from build123d import *

# Parameters (mm, degrees)
F0_R     = 1.45
F1_DEPTH = 7.62
F2_R     = 1.877804
F3_DEPTH = 25.4
F5_W     = 7.426485
F5_H     = 4.44201
F6_DEPTH = 25.4


with BuildPart() as f1:
    # F0 (on Right) → F1 (new body)
    with BuildSketch(Plane.YZ):
        with Locations((0, 11.320898)):
            Circle(F0_R)
    extrude(amount=F1_DEPTH)

    # F2 (on Top) → F3 (join)
    with BuildSketch(Plane.XY):
        with Locations((-1.127225, 0)):
            Circle(F2_R)
    extrude(amount=F3_DEPTH)

    # F5 (on offset) → F6 (join)
    with BuildSketch(Plane.XY.offset(17.78)):
        with Locations((-1.208354, -0.011814)):
            Rectangle(F5_W, F5_H)
    extrude(amount=F6_DEPTH)


solid = f1.part
Check sheet for the modelled part. Datum: model origin and axes. Units: mm. A direction names the side the tool comes from. Round coordinates to 2 decimals unless told otherwise and drop trailing zeros. Order: outer loops, then holes, each group sorted by start corner. A loop starts at its lowest first (then second) coordinate and runs counter-clockwise, first axis right, second up.
(1) Cross-section at C-C, the plane z = 37. Enter the section's corners in (x, y).
(2) Cross-section at A-A, the plane y = 0. Enter the section's corners in (x, z).
(3) Scan lines: probe 1 along X at (y, z) = (0.5, 22); probe 2 along Z at (x, y) = (1, 1); probe 3 along Z at (x, y) = (-4, -0.35). Record each from-to range of solid material in increasing order.
(4) Cross-section at B-B, the plane x = 1.25. Enter the section's corners in (y, z).
(5) Cross-section at D-D, the plane x = 6. Enter the section's corners in (y, z), and give its area (3 significant figures).
(6) Access from +Z, -Z, +X, -X, +Y, -Y to the whole of each face (thin tool, end or side, straight path). Record for faces 1 (the flat face through (2.505, 0, 30)), 2 (the flat face through (-1, 0, 0)).
(7) Draft check along Z on faces 3 (the flat face through (7.62, 0, 11)), 4 (the cylindrical face through (3.79, -1.45, 11.38)), 5 (the flat face through (-3, -1, 17.78)), 6 (the flat face through (-1, 0, 43.18)). Enter one of: pulls with the +Z half, pulls with the -Z half, needs draft (parallel to the pull), parting line crosses it, or undercut.
(8) Go/stop test with a flat-tipped pin: P1, Ø6, axis at x = -3, z = 8, coming from the -Y side. Record where the tip stops, or that it passes through.
Check sheet entries:
1. outline: (-4.92, -2.23) - (2.5, -2.23) - (2.5, 2.21) - (-4.92, 2.21) - close
2. outline: (-4.92, 17.78) - (-3.01, 17.78) - (-3.01, 0) - (0.75, 0) - (0.75, 9.87) - (7.62, 9.87) - (7.62, 12.77) - (0.75, 12.77) - (0.75, 17.78) - (2.5, 17.78) - (2.5, 43.18) - (-4.92, 43.18) - close
3. probe 1: x = -4.92 to 2.5
3. probe 2: z = 10.27 to 12.37, 17.78 to 43.18
3. probe 3: z = 17.78 to 43.18
4. outline: (-2.23, 17.78) - (2.21, 17.78) - (2.21, 43.18) - (-2.23, 43.18) - close; circle Ø2.9 at (0, 11.32)
5. outline: circle Ø2.9 at (0, 11.32)
5. area: 6.61 mm2
6. face 1: +Z, +X, +Y, -Y
6. face 2: -Z, +X, -X, +Y, -Y
7. face 3: needs draft
7. face 4: undercut
7. face 5: undercut
7. face 6: pulls with the +Z half
8. P1: stops at y = -1.88
